Could you check a few things on this model? Use its own coordinates, in mm. A direction names the side the tool comes from. Round coordinates to 2 decimals unless told otherwise and drop trailing zeros. Write each loop counter-clockwise with the first axis right and the second up, starting at its lowest first coordinate (ties: lowest second). Pieces come first, ordered by that corner, then holes. Notation, with made-up numbers: M 48.5,-14.5 L 63.5,-14.5 A15 ccw 63.5,0.5 Z; hole C -6,5 d1. An arc over 180 degrees is marked long. One line per item, written item: value. Start each with the question number.
(1) I want a section at B-B on x = 8. Please give me the cut outline in (y, z), and give its area (3 significant figures).
(2) Which directions (+Z, -Z, +X, -X, +Y, -Y) give clear straight access to the entire face, cutting with the end or side of a thin tool? Please do faces 4 (the face through (-0.867, -43.651, -3.905)), 5 (the face through (-0.867, 43.651, -3.905)), 6 (the face through (13.4, -32.5, 7.5)).
(3) If I drill on L1, parallel to Z at x = -36, y = 0; L2, parallel to Y at x = 9.5, z = 2.75; L3, parallel to X at y = 16.5, z = 4.75, over which ranges is the centre line in solid material (lowest first)?
(4) I want a section at A-A on z = 0. Please give me the cut outline in (x, y).
(5) I want a section at D-D on y = 0. Please give me the cut outline in (x, z).
(6) I want a section at C-C on y = -15. Please give me the cut outline in (x, z).
(7) Thinking about a two-plate mould opening in Y: for faces 1 (the face through (-36.266, -0.867, -3.905)), 2 (the face through (-13.4, -32.5, -7.5)), 3 (the face through (36.266, -0.867, -3.905)), which applies, released by +Y, released by -Y, zero draft, split by the parting line, or undercut?
(8) I'm going to push flat-ended pins straight in: pin 1 Ø9 at (y, z) = (0, 0) entering from +X; pin 2 Ø2 at (y, z) = (3.5, -4.5) entering from -X; pin 3 Ø5 at (x, z) = (-5.5, 0.5) entering from +Y; pin 4 Ø4 at (y, z) = (33.5, 2) entering from -X. Where does each tip first touch, or does it pass through?
```python
from build123d import *

# Parameters (mm, degrees)
F2_R          = 4
F3_DEPTH      = 37.501
F3_DEPTH_BACK = 37.501
F5_R          = 4


with BuildPart() as f1:
    # F0 (on Front) → F1 (revolve)
    with BuildSketch(Plane.XZ):
        with BuildLine():
            Line((-34.6987031458, 7.5), (-36.7423461417, 7.5))
            ThreePointArc((-36.7423461417, 7.5), (-37.5, 0), (-36.7423461417, -7.5))
            Line((-36.7423461417, -7.5), (-34.6987031458, -7.5))
            ThreePointArc((-34.6987031458, -7.5), (-35.5, 0), (-34.6987031458, 7.5))
        make_face()
    revolve(axis=Axis((0, 0, 16.8621425897), (0, 0, -1)))

    # F2 (on Right) → F3 (cut, two sides)
    with BuildSketch(Plane.YZ) as f3_sk:
        Circle(F2_R)
    extrude(amount=-F3_DEPTH, mode=Mode.SUBTRACT)
    extrude(f3_sk.sketch, amount=F3_DEPTH_BACK, mode=Mode.SUBTRACT)

    # F5 (on offset) → F6 (join, up to the next surface of F1)
    with BuildSketch(Plane.XZ.offset(50)):
        Circle(F5_R)
    extrude(until=Until.NEXT, dir=(0, 1, 0))

    # F7: F1 across plane


with BuildPart() as f1_1:
    add(f1.part)
    add(f1.part.mirror(Plane.XZ))

    # F8 (on Right) → F9 (revolve, cut)
    with BuildSketch(Plane.YZ):
        with BuildLine():
            Line((0, 50), (0, 55))
            ThreePointArc((0, 55), (-55, 0), (0, -55))
            Line((0, -55), (0, -50))
            ThreePointArc((0, -50), (-50, 0), (0, 50))
        make_face()
    revolve(axis=Axis((0, 0, 27.5), (0, 0, -1)), mode=Mode.SUBTRACT)


solid = f1_1.part
```
Found:
1. outline: M -35.86,-7.5 L -33.76,-7.5 A34.59 cw -33.76,7.5 L -35.86,7.5 A36.64 ccw Z; M 33.76,-7.5 L 35.86,-7.5 A36.64 ccw 35.86,7.5 L 33.76,7.5 A34.59 cw Z
1. area: 62.0 mm²
2. face 4: -Y
2. face 5: +Y
2. face 6: +Z, +X, -X, +Y, -Y
3. L1: z = -7.5 to -4, 4 to 7.5
3. L2: y = -36.17 to -34.09, 34.09 to 36.17
3. L3: x = -33.34 to -31.07, 31.07 to 33.34
4. outline: M -37.29,-4 A37.5 ccw -4,-37.29 L -4,-49.84 A50 ccw 4,-49.84 L 4,-37.29 A37.5 ccw 37.29,-4 L 35.27,-4 A35.5 cw -35.27,-4 Z; M -37.29,4 L -35.27,4 A35.5 cw 35.27,4 L 37.29,4 A37.5 ccw 4,37.29 L 4,49.84 A50 ccw -4,49.84 L -4,37.29 A37.5 ccw Z
5. outline: M -37.29,-4 A37.5 ccw -36.74,-7.5 L -34.7,-7.5 A35.5 cw -35.27,-4 Z; M -37.29,4 L -35.27,4 A35.5 cw -34.7,7.5 L -36.74,7.5 A37.5 ccw Z; M 34.7,-7.5 L 36.74,-7.5 A37.5 ccw 37.29,-4 L 35.27,-4 A35.5 cw Z; M 34.7,7.5 A35.5 cw 35.27,4 L 37.29,4 A37.5 ccw 36.74,7.5 Z
6. outline: M -33.54,-7.5 L -31.29,-7.5 A32.18 cw -31.29,7.5 L -33.54,7.5 A34.37 ccw Z; M 31.29,-7.5 L 33.54,-7.5 A34.37 ccw 33.54,7.5 L 31.29,7.5 A32.18 cw Z
7. face 1: undercut
7. face 2: zero draft
7. face 3: undercut
8. pin 1: stops at x = 37.29
8. pin 2: stops at x = -37.2
8. pin 3: stops at y = 49.91
8. pin 4: stops at x = -20.25
